Input: part model. Units: mm. Frame: model coordinates. Face numbers are marked on the shaded views. Coordinates: 2 decimals unless noted, no trailing zeros. Loops run counter-clockwise (first coordinate to the right, second up) from the corner with the lowest first, then second, coordinate; pieces in that order, holes last.
```python
from build123d import *

# Parameters (mm, degrees)
F10_R     = 6.35
F15_DEPTH = 67.174456
F11_R     = 6.35
F16_DEPTH = 67.174457
F14_R     = 6.35
F17_DEPTH = 50.739447
F13_R     = 6.35
F18_DEPTH = 50.739447
F9_R      = 6.35
F19_DEPTH = 67.174457
F12_R     = 6.35
F20_DEPTH = 67.174457
F21_D     = 9.525


with BuildPart() as f1:
    # F0 (on Front) → F1 (revolve)
    with BuildSketch(Plane.XZ):
        Polygon((-8.255, 0), (0, 0), (0, 12.7), (20.32, 33.02), (20.32, 43.18), (0, 63.5), (-8.255, 63.5), align=None)
    revolve(axis=Axis((-4.1275, 0, 0), (1, 0, 0)))

    # F10 (on face) → F15 (cut, through all)
    with BuildSketch(Plane(origin=(0, 0, 0), x_dir=(-0.267261, 0.935414, 0.231455), z_dir=(0.707107, 0.353553, -0.612372))):
        with Locations((-10.800335, 26.455309)):
            Circle(F10_R)
    extrude(amount=-F15_DEPTH, mode=Mode.SUBTRACT)

    # F11 (on face) → F16 (cut, through all)
    with BuildSketch(Plane(origin=(0, 0, 0), x_dir=(0.267261, 0.935414, -0.231455), z_dir=(0.707107, -0.353553, -0.612372))):
        with Locations((10.800335, 26.455309)):
            Circle(F11_R)
    extrude(amount=-F16_DEPTH, mode=Mode.SUBTRACT)

    # F14 (on face) → F17 (cut, through all)
    with BuildSketch(Plane(origin=(0, 0, 0), x_dir=(-0.707107, 0.707107, 0), z_dir=(0.707107, 0.707107, 0))):
        with Locations((-28.575, 0)):
            Circle(F14_R)
    extrude(amount=-F17_DEPTH, mode=Mode.SUBTRACT)

    # F13 (on face) → F18 (cut, through all)
    with BuildSketch(Plane(origin=(0, 0, 0), x_dir=(-0.707107, -0.707107, 0), z_dir=(-0.707107, 0.707107, 0))):
        with Locations((-28.575, 0)):
            Circle(F13_R)
    extrude(amount=F18_DEPTH, mode=Mode.SUBTRACT)

    # F9 (on face) → F19 (cut, through all)
    with BuildSketch(Plane(origin=(0, 0, 0), x_dir=(0.267261, 0.935414, 0.231455), z_dir=(0.707107, -0.353553, 0.612372))):
        with Locations((10.800335, -26.455309)):
            Circle(F9_R)
    extrude(amount=-F19_DEPTH, mode=Mode.SUBTRACT)

    # F12 (on face) → F20 (cut, through all)
    with BuildSketch(Plane(origin=(0, 0, 0), x_dir=(-0.267261, 0.935414, -0.231455), z_dir=(0.707107, 0.353553, 0.612372))):
        with Locations((-10.800335, -26.455309)):
            Circle(F12_R)
    extrude(amount=-F20_DEPTH, mode=Mode.SUBTRACT)

    # F21 (through all)
    with Locations(Plane.YZ):
        with Locations((0, 0)):
            Hole(F21_D / 2)


solid = f1.part
```
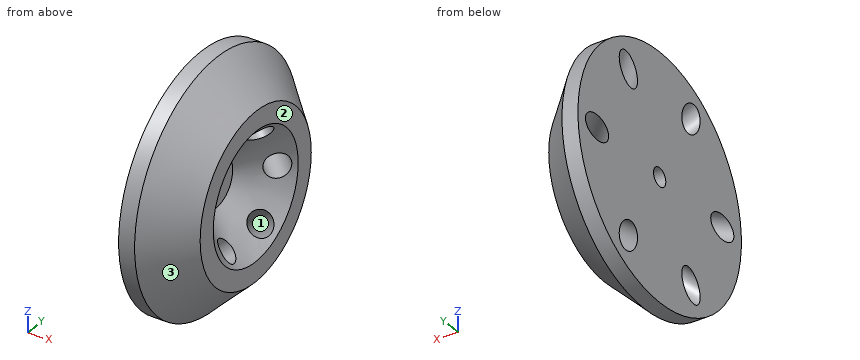
Item 1: Section query A-A (y = 0). Output: boundary loops of the cut face in (x, z) (1 decimal).
Result:
outline: (-8.3, -63.5) - (0, -63.5) - (20.3, -43.2) - (20.3, -33) - (0, -12.7) - (0, -4.8) - (-8.3, -4.8) - close; (-8.3, 4.8) - (0, 4.8) - (0, 12.7) - (20.3, 33) - (20.3, 43.2) - (0, 63.5) - (-8.3, 63.5) - close
Item 2: Line query: L1, parallel to Z at x = -3.5, y = 0; L2, parallel to Y at x = 9, z = -31; L3, parallel to X at y = 16.5, z = 48 (3 decimals). Output: solid intervals per line, ascending.
Result:
L1: z = -63.5 to -4.76, 4.76 to 63.5
L2: y = -44.82 to -22.7, -10.59 to 10.59, 22.7 to 44.82
L3: x = -8.255 to 12.743
Item 3: Mould query, pull axis Y, two halves, no side actions, for the marked faces 1, 2 and 3. Classes: +Y half, -Y half, draft (parallel to the pull), parting line (faces both ways), or undercut.
Result:
face 1: undercut
face 2: draft
face 3: parting line
Item 4: Section query C-C (x = 3.5). Count the separate pieces of the cut face and the enclosed holes in it, then the cut area to 3 significant figures.
Result:
separate pieces: 1
enclosed holes: 7
area: 9,410 mm2
Item 5: Section query B-B (z = 0). Output: boundary loops of the cut face in (x, y) (1 decimal).
Result:
outline: (-8.3, -63.5) - (0, -63.5) - (20.3, -43.2) - (20.3, -33) - (18.3, -31) - (-8.3, -57.6) - close; (-8.3, -39.7) - (9.4, -22.1) - (0, -12.7) - (0, -4.8) - (-8.3, -4.8) - close; (-8.3, 4.8) - (0, 4.8) - (0, 12.7) - (9.4, 22.1) - (-8.3, 39.7) - close; (-8.3, 57.6) - (18.3, 31) - (20.3, 33) - (20.3, 43.2) - (0, 63.5) - (-8.3, 63.5) - close
Item 6: Contact query for flat-ended pins moving along their axis: P1, Ø10, axis at x = 5, z = 22.5, coming from the +Y side; P2, Ø1, axis at x = -5, y = 5, coming from the -Z side; P3, Ø7.5, axis at y = 0, z = 0, coming from the -X side; P4, Ø1.5, axis at y = -13.5, z = 41.5, coming from the +X side. Output: stop coordinate, or through.
Result:
P1: stops at y = 59.68
P2: stops at z = -63.34
P3: passes through
P4: stops at x = 20.32
